Check sheet for the modelled part. Datum: model origin and axes. Units: mm. A direction names the side the tool comes from. Give positions to 0.01 mm unless a question says otherwise; leave off trailing zeros. Order: outer loops, then holes, each group sorted by start corner. A loop starts at its lowest first (then second) coordinate and runs counter-clockwise, first axis right, second up.
Item 1: Sectioned sample at B-B on z = 6.35. Record the boundary of the cut face in (x, y).
Item 2: Sectioned sample at A-A on x = -12.7. Record the boundary of the cut face in (y, z) (3 decimals).
Item 3: Sectioned sample at C-C on x = 39.5. Record the boundary of the cut face in (y, z) (3 decimals), and give its area (3 significant figures).
Item 4: Material ranges on line 1 along X through (y, z) = (3.35, -19.05); line 2 along X through (y, z) = (3.75, -6.35); line 3 along Z through (x, y) = (37, 1.1) (3 decimals), recorded low to high.
Item 5: Gauge pin test, flat ends, axial feed: P1, Ø0.8, axis at y = 4.5, z = 1.5, coming from the -X side; P2, Ø1.4, axis at x = 36.83, z = 19.05, coming from the -Y side; P3, Ø16.5, axis at x = 36, z = 5, coming from the +Y side. Record the tip position at first contact, or that the pin passes through.
Item 6: Access from +Z, -Z, +X, -X, +Y, -Y to the whole of each face (thin tool, end or side, straight path). Record for faces 1 (the flat face through (35, 2.54, 0)), 2 (the flat face through (-17, 4.064, 0)), 3 (the cylindrical face through (47.28, 2.58, 19.87)).
Item 7: Release check for a two-part mould opening along X. For faces 4 (the flat face through (8, 3, 22.225)), 5 (the flat face through (35, 4, -16.5)), 6 (the flat face through (-33.02, 2, 0)) record: released by +X, released by -X, zero draft, split by the parting line, or undercut.
Item 8: Sectioned sample at D-D on x = 12.7. Record the boundary of the cut face in (y, z) (1 decimal), and give its area (3 significant figures).
from build123d import *

# Parameters (mm, degrees)
SKETCH1_W           = 101.6
SKETCH1_H           = 44.45
BOSS_EXTRUDE1_DEPTH = 5.08
SKETCH2_R           = 0.889
CUT_EXTRUDE1_DEPTH  = 56.681208904
SKETCH3_R           = 1.2192
SKETCH3_R_2         = 1.5875
CUT_EXTRUDE2_DEPTH  = 56.681208904
SKETCH4_W           = 17.78
SKETCH4_H           = 34.036
CUT_EXTRUDE3_DEPTH  = 56.681208904
FILLET2_R           = 2.54
SKETCH5_W           = 17.78
SKETCH5_H           = 44.45
CUT_EXTRUDE4_DEPTH  = 56.681208904
SKETCH6_W           = 33.02
SKETCH6_H           = 33.02
CUT_EXTRUDE5_DEPTH  = 1.016
FILLET3_R           = 1.27
SKETCH7_W           = 20.32
SKETCH7_H           = 33
CUT_EXTRUDE6_DEPTH  = 2.54
FILLET4_R           = 1.27


with BuildPart() as part:
    # Sketch1 → Boss-Extrude1 (new body)
    with BuildSketch(Plane(origin=(0, 0, 0), x_dir=(1, 0, 0), z_dir=(0, 1, 0))):
        Rectangle(SKETCH1_W, SKETCH1_H)
    extrude(amount=BOSS_EXTRUDE1_DEPTH)

    # Sketch2 → Cut-Extrude1 (cut, through all)
    with BuildSketch(Plane(origin=(0, 5.08, 0), x_dir=(1, 0, 0), z_dir=(0, 1, 0))):
        with Locations(Location((-46.99, 19.05, 0), (0, 0, 270))):
            Circle(SKETCH2_R)
        with Locations(Location((-29.21, 19.05, 0), (0, 0, 270))):
            Circle(SKETCH2_R)
        with Locations(Location((-12.7, 19.05, 0), (0, 0, 270))):
            Circle(SKETCH2_R)
        with Locations(Location((25.4, 19.05, 0), (0, 0, 270))):
            Circle(SKETCH2_R)
        with Locations(Location((36.83, 19.05, 0), (0, 0, 270))):
            Circle(SKETCH2_R)
        with Locations(Location((47.625, 19.05, 0), (0, 0, 270))):
            Circle(SKETCH2_R)
        with Locations(Location((47.625, 0, 0), (0, 0, 270))):
            Circle(SKETCH2_R)
        with Locations(Location((47.625, -19.05, 0), (0, 0, 270))):
            Circle(SKETCH2_R)
        with Locations(Location((36.83, -19.05, 0), (0, 0, 270))):
            Circle(SKETCH2_R)
        with Locations(Location((25.4, -19.05, 0), (0, 0, 270))):
            Circle(SKETCH2_R)
        with Locations(Location((-12.7, -19.05, 0), (0, 0, 270))):
            Circle(SKETCH2_R)
        with Locations(Location((-29.21, -19.05, 0), (0, 0, 270))):
            Circle(SKETCH2_R)
        with Locations(Location((-46.99, -19.05, 0), (0, 0, 270))):
            Circle(SKETCH2_R)
        with Locations(Location((19.05, -6.35, 0), (0, 0, 270))):
            Circle(SKETCH2_R)
        with Locations(Location((19.05, 6.35, 0), (0, 0, 270))):
            Circle(SKETCH2_R)
        with Locations(Location((6.35, 6.35, 0), (0, 0, 270))):
            Circle(SKETCH2_R)
        with Locations(Location((6.35, -6.35, 0), (0, 0, 270))):
            Circle(SKETCH2_R)
    extrude(amount=-CUT_EXTRUDE1_DEPTH, mode=Mode.SUBTRACT)

    # Sketch3 → Cut-Extrude2 (cut, through all)
    with BuildSketch(Plane(origin=(0, 5.08, 0), x_dir=(1, 0, 0), z_dir=(0, 1, 0))):
        with Locations(Location((-37.846, 19.3294, 0), (0, 0, 270))):
            Circle(SKETCH3_R)
        with Locations(Location((12.7, 15.875, 0), (0, 0, 270))):
            Circle(SKETCH3_R_2)
    cut_extrude2 = extrude(amount=-CUT_EXTRUDE2_DEPTH, mode=Mode.SUBTRACT)

    # Mirror1: Cut-Extrude2 across plane
    add(cut_extrude2.mirror(Plane.XY), mode=Mode.SUBTRACT)

    # Sketch4 → Cut-Extrude3 (cut, through all)
    with BuildSketch(Plane(origin=(0, 5.08, 0), x_dir=(1, 0, 0), z_dir=(0, 1, 0))):
        with Locations((-41.91, 0)):
            Rectangle(SKETCH4_W, SKETCH4_H)
    extrude(amount=-CUT_EXTRUDE3_DEPTH, mode=Mode.SUBTRACT)

    # Fillet2
    fillet2_edges = [part.edges().sort_by_distance(p)[0] for p in [
        (-33.02, 2.54, -17.018),
        (-33.02, 2.54, 17.018),
    ]]
    fillet(fillet2_edges, radius=FILLET2_R)

    # Sketch5 → Cut-Extrude4 (cut, through all)
    with BuildSketch(Plane(origin=(0, 5.08, 0), x_dir=(1, 0, 0), z_dir=(0, 1, 0))):
        with Locations((-41.91, 0)):
            Rectangle(SKETCH5_W, SKETCH5_H)
    extrude(amount=-CUT_EXTRUDE4_DEPTH, mode=Mode.SUBTRACT)

    # Sketch6 → Cut-Extrude5 (cut)
    with BuildSketch(Plane(origin=(0, 5.08, 0), x_dir=(1, 0, 0), z_dir=(0, 1, 0))):
        with Locations((-16.51, 0)):
            Rectangle(SKETCH6_W, SKETCH6_H)
    extrude(amount=-CUT_EXTRUDE5_DEPTH, mode=Mode.SUBTRACT)

    # Fillet3
    fillet3_edges = [part.edges().sort_by_distance(p)[0] for p in [
        (0, 4.572, -16.51),
        (0, 4.572, 16.51),
    ]]
    fillet(fillet3_edges, radius=FILLET3_R)

    # Sketch7 → Cut-Extrude6 (cut)
    with BuildSketch(Plane(origin=(0, 5.08, 0), x_dir=(1, 0, 0), z_dir=(0, 1, 0))):
        with Locations((35.56, 0)):
            Rectangle(SKETCH7_W, SKETCH7_H)
    extrude(amount=-CUT_EXTRUDE6_DEPTH, mode=Mode.SUBTRACT)

    # Fillet4
    fillet4_edges = [part.edges().sort_by_distance(p)[0] for p in [
        (45.72, 3.81, -16.5),
        (45.72, 3.81, 16.5),
        (25.4, 3.81, 16.5),
        (25.4, 3.81, -16.5),
    ]]
    fillet(fillet4_edges, radius=FILLET4_R)


solid = part.part
Report:
1. outline: (-33.02, 0) - (5.46, 0) - (5.46, 5.08) - (0, 5.08) - (0, 4.06) - (-33.02, 4.06) - close; (7.24, 0) - (18.16, 0) - (18.16, 5.08) - (7.24, 5.08) - close; (19.94, 0) - (50.8, 0) - (50.8, 5.08) - (45.72, 5.08) - (45.72, 2.54) - (25.4, 2.54) - (25.4, 5.08) - (19.94, 5.08) - close
2. outline: (0, -22.225) - (5.08, -22.225) - (5.08, -19.939) - (0, -19.939) - close; (0, -18.161) - (5.08, -18.161) - (5.08, -16.51) - (4.064, -16.51) - (4.064, 16.51) - (5.08, 16.51) - (5.08, 18.161) - (0, 18.161) - close; (0, 19.939) - (5.08, 19.939) - (5.08, 22.225) - (0, 22.225) - close
3. outline: (0, -22.225) - (5.08, -22.225) - (5.08, -16.5) - (2.54, -16.5) - (2.54, 16.5) - (5.08, 16.5) - (5.08, 22.225) - (0, 22.225) - close
3. area: 142 mm2
4. line 1: x = -33.02 to -30.1, -28.32 to -13.59, -11.81 to 24.51, 26.29 to 35.94, 37.72 to 46.74, 48.51 to 50.8
4. line 2: x = -33.02 to 5.46, 7.24 to 18.16, 19.94 to 25.4, 45.72 to 50.8
4. line 3: z = -22.225 to -19.923, -18.177 to 18.177, 19.923 to 22.225
5. P1: stops at x = 0
5. P2: passes through
5. P3: stops at y = 2.54
6. face 1: +Y
6. face 2: -X, +Y
6. face 3: +Y, -Y
7. face 4: zero draft
7. face 5: undercut
7. face 6: released by -X
8. outline: (0, -22.2) - (5.1, -22.2) - (5.1, -17.5) - (0, -17.5) - close; (0, -14.3) - (5.1, -14.3) - (5.1, 14.3) - (0, 14.3) - close; (0, 17.5) - (5.1, 17.5) - (5.1, 22.2) - (0, 22.2) - close
8. area: 194 mm2
